from build123d import *

# Parameters (mm, degrees)
SKETCH1_W           = 100
SKETCH1_H           = 80
BOSS_EXTRUDE1_DEPTH = 1.5
FILLET1_R           = 2
SKETCH7_W           = 30
SKETCH7_H           = 30
BUKAAN_DEPTH        = 7.5
SKETCH8_W           = 26.5
SKETCH8_H           = 15.5
CUT_EXTRUDE6_DEPTH  = 10.5


with BuildPart() as part:
    # Sketch1 → Boss-Extrude1 (new body)
    with BuildSketch(Plane(origin=(0, 0, 0), x_dir=(1, 0, 0), z_dir=(0, 1, 0))):
        with Locations((22.937293729, 8.811881188)):
            Rectangle(SKETCH1_W, SKETCH1_H)
    extrude(amount=BOSS_EXTRUDE1_DEPTH)

    # Fillet1
    fillet1_edges = [part.edges().sort_by_distance(p)[0] for p in [
        (-27.062706271, 0.75, -48.811881188),
        (72.937293729, 0.75, -48.811881188),
        (72.937293729, 0.75, 31.188118812),
        (-27.062706271, 0.75, 31.188118812),
    ]]
    fillet(fillet1_edges, radius=FILLET1_R)

    # Sketch7 → bukaan (cut)
    with BuildSketch(Plane(origin=(0, 1.5, 0), x_dir=(1, 0, 0), z_dir=(0, 1, 0))):
        with Locations((-1.545768262, 33.811881188)):
            Rectangle(SKETCH7_W, SKETCH7_H)
    extrude(amount=-BUKAAN_DEPTH, mode=Mode.SUBTRACT)

    # Sketch8 → Cut-Extrude6 (cut)
    with BuildSketch(Plane(origin=(0, 0, 0), x_dir=(1, 0, 0), z_dir=(0, 1, 0))):
        with Locations((48.400499743, 33.583205548)):
            Rectangle(SKETCH8_W, SKETCH8_H)
    extrude(amount=CUT_EXTRUDE6_DEPTH, mode=Mode.SUBTRACT)


solid = part.part
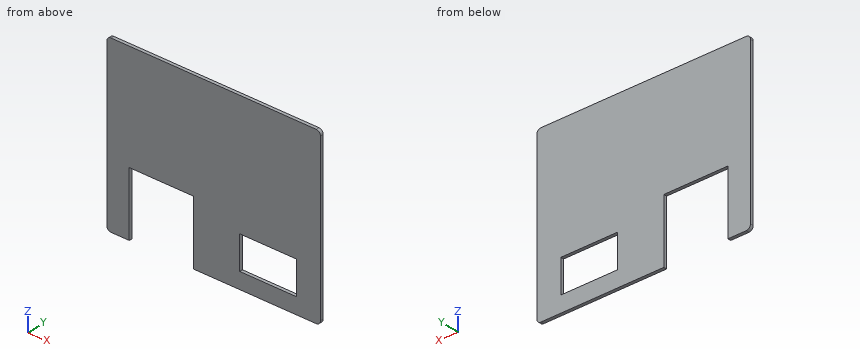
Input: part model. Units: mm. Frame: model coordinates. Coordinates: 2 decimals unless noted, no trailing zeros. Loops run counter-clockwise (first coordinate to the right, second up) from the corner with the lowest first, then second, coordinate; pieces in that order, holes last.
Q1. Contact query for a flat-ended pin moving along its axis: pin 1 (0.8 mm diameter, centred on x = 1.5, y = 0.5, fed in from -Z). Output: stop coordinate, or through.
Q2. Material intervals for line 1 (X direction, y = 0.6, z = -31); line 2 (Z direction, x = 37, y = 1.2); line 3 (Z direction, x = 2, y = 0.7), sorted ascending.
Q3. Cut plane A-A (x = 56). Output: boundary loops of the cut face in (y, z), then the cut area to 4 significant figures.
Q4. Cut plane C-C (x = 3.5). Output: boundary loops of the cut face in (y, z).
Q5. Cut plane B-B (y = 0.8). Output: boundary loops of the cut face in (x, z), then the cut area to 3 significant figures.
Working result:
1. pin 1: stops at z = -18.81
2. line 1: x = -27.06 to -16.55, 13.45 to 35.15, 61.65 to 72.94
2. line 2: z = -48.81 to -41.33, -25.83 to 31.19
2. line 3: z = -18.81 to 31.19
3. outline: (0, -48.81) - (1.5, -48.81) - (1.5, -41.33) - (0, -41.33) - close; (0, -25.83) - (1.5, -25.83) - (1.5, 31.19) - (0, 31.19) - close
3. area: 96.75 mm2
4. outline: (0, -18.81) - (1.5, -18.81) - (1.5, 31.19) - (0, 31.19) - close
5. outline: (-27.06, -46.81) arc R2 ccw to (-25.06, -48.81) - (-16.55, -48.81) - (-16.55, -18.81) - (13.45, -18.81) - (13.45, -48.81) - (70.94, -48.81) arc R2 ccw to (72.94, -46.81) - (72.94, 29.19) arc R2 ccw to (70.94, 31.19) - (-25.06, 31.19) arc R2 ccw to (-27.06, 29.19) - close; hole (35.15, -41.33) - (61.65, -41.33) - (61.65, -25.83) - (35.15, -25.83) - close
5. area: 6,690 mm2
